Design review of the part built by this model. Coordinates are the model's own, in mm. Face numbers are marked on the shaded views. Give positions to 0.01 mm unless a question says otherwise; leave off trailing zeros. Loops run counter-clockwise (first coordinate to the right, second up) from the corner with the lowest first, then second, coordinate; pieces in that order, holes last. Notation, with made-up numbers: (37, -17) -> (45, -17) arc R9 ccw to (45, 0) -> close; hole circle Ø2 at (-22.75, 42). An arc over 180 degrees is marked (long way). Use CSV: the item, a comma, the result in double quotes. Start each with the question number.
Item 1: Clearance check with flat-ended pins moving along their axes: pin 1 (1.5 mm diameter, centred on x = 2, z = 8.5, fed in from +Y); pin 2 (2 mm diameter, centred on x = -0.5, z = 14, fed in from +Y); pin 3 (1.5 mm diameter, centred on y = 2, z = 9.5, fed in from -X); pin 4 (3 mm diameter, centred on x = 0.5, z = 6.5, fed in from -Y). State where each tip first meets the part, or that it passes through.
Item 2: We need section C-C (z = 8.75). State the section outline as (x, y) points, plus the area to 3 significant figures.
Item 3: We need section A-A (z = 3.5). State the section outline as (x, y) points.
Item 4: Wall thickness on line 1 along Y through (x, z) = (1, 11.75); line 2 along Z through (x, y) = (1, 1.25); line 3 along Y through (x, z) = (0.75, 4.5): over which ranges is each line inside the solid? List them lowest first. Write a range as from..to.
Item 5: We need section D-D (z = 13.75). State the section outline as (x, y) points.
Item 6: The part is to be moulded in two halves that separate along Y. For the marked faces 1, 2 and 3, say which applies: +Y half, -Y half, draft (parallel to the pull), parting line (faces both ways), or undercut.
from build123d import *

# Parameters (mm, degrees)
F0_R          = 3.5
F1_DEPTH      = 6
F1_FACE_R     = 3.5
F2_DEPTH      = 15
F2_TAPER      = 1
F3_W          = 4
F3_H          = 4
F4_DEPTH      = 18.45601
F5_W          = 1.5
F5_H          = 7
F6_DEPTH      = 3.501
F6_DEPTH_BACK = 3.501
F7_R          = 0.5


with BuildPart() as f1:
    # F0 (on Top) → F1 (new body)
    with BuildSketch(Plane.XY):
        Circle(F0_R)
    extrude(amount=F1_DEPTH)

    # F1_face (on face) → F2 (join)
    with BuildSketch(Plane.XY.offset(6)):
        Circle(F1_FACE_R)
    extrude(amount=F2_DEPTH, taper=F2_TAPER)

    # F3 (on face) → F4 (cut)
    with BuildSketch(Plane(origin=(0, 0, 0), x_dir=(1, 0, 0), z_dir=(0, 0, -1))):
        Rectangle(F3_W, F3_H)
    extrude(amount=-F4_DEPTH, mode=Mode.SUBTRACT)

    # F5 (on Right) → F6 (cut, two sides)
    with BuildSketch(Plane.YZ) as f6_sk:
        with Locations((0, 3.5)):
            Rectangle(F5_W, F5_H)
    extrude(amount=-F6_DEPTH, mode=Mode.SUBTRACT)
    extrude(f6_sk.sketch, amount=F6_DEPTH_BACK, mode=Mode.SUBTRACT)

    # F7
    f7_edges = [f1.edges().sort_by_distance(p)[0] for p in [
        (-3.238174, 0, 21),
    ]]
    fillet(f7_edges, radius=F7_R)


solid = f1.part
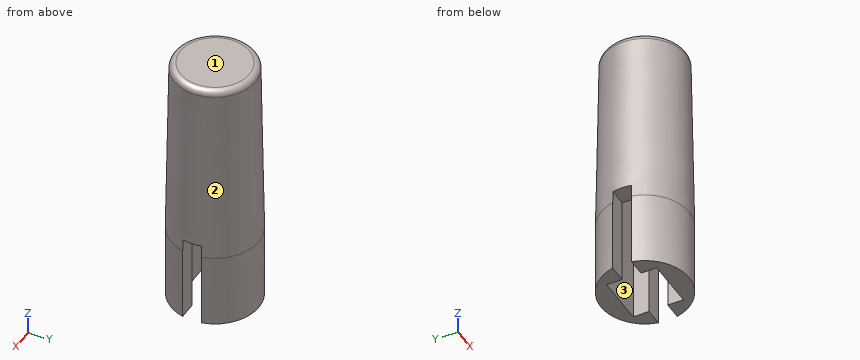
Results found:
1,pin 1,"y = 3.22"
1,pin 2,"y = 3.38"
1,pin 3,"x = -3.2"
1,pin 4,"y = -3.5"
2,outline,"circle Ø6.9 at (0, 0); hole (-2, -2) -> (2, -2) -> (2, 2) -> (-2, 2) -> close"
2,area,"21.4 mm²"
3,outline,"(-3.42, -0.75) arc R3.5 ccw to (3.42, -0.75) -> (2, -0.75) -> (2, -2) -> (-2, -2) -> (-2, -0.75) -> close; (-3.42, 0.75) -> (-2, 0.75) -> (-2, 2) -> (2, 2) -> (2, 0.75) -> (3.42, 0.75) arc R3.5 ccw to start"
4,line 1,"-3.25..-2, 2..3.25"
4,line 2,"18.46..21"
4,line 3,"-3.42..-2, 2..3.42"
5,outline,"circle Ø6.73 at (0, 0); hole (-2, -2) -> (2, -2) -> (2, 2) -> (-2, 2) -> close"
6,face 1,"draft"
6,face 2,"parting line"
6,face 3,"undercut"
